Autodesk Inventor part; units mm, degrees
ref_plane "YZ Plane" through (0, 0, 0) normal (1, 0, 0) x (0, 1, 0)
ref_plane "XZ Plane" through (0, 0, 0) normal (0, 1, 0) x (-1, 0, 0)
ref_plane "XY Plane" through (0, 0, 0) normal (0, 0, 1) x (1, 0, 0)
sketch "Skizze1" plane through (0, 0, 0) normal (0, 1, 0) x (-1, 0, 0)
  line L0 (0, 0) -> (0, 79.9753) construction
  line L1 (0, 0) -> (-80.4332, 0) construction
  line L2 (0, 0) -> (80.1339, 0) construction
  line L3 (0, 0) -> (0, -79.3949) construction
  line L4 (0, 1.55) -> (-17, 1.55)
  line L5 (-17, 1.55) -> (-17, 2.95)
  line L6 (-17, 2.95) -> (0, 2.95)
  arc A0 (-1.3565, 0.75) -> (0, 1.55) centre (0, 0) ccw
  arc A1 (-2.8531, 0.75) -> (0, 2.95) centre (0, 0) ccw
  line L7 (-1.3565, 0.75) -> (-2.8531, 0.75)
  circle A2 centre (0, 0) radius 1.5
  dimension "d0" = 1.4
  dimension "d1" = 5.9
  dimension "d2" = 0.8
  dimension "d3" = 19.95
  dimension "d21" = 0.05
  dimension "d28" = 17
extrude "Extrusion1" add sketch "Skizze1" along normal mid plane 60 contours L4 L5 L6 A1 L7 A0
sketch "Skizze3" plane through (0, 0, 0) normal (0, 0, 1) x (1, 0, 0)
  line L0 (7.5, -7.25) -> (-7, -7.25)
  line L1 (-7, -7.25) -> (-7, 7.25)
  line L2 (-7, 7.25) -> (7.5, 7.25)
  line L3 (7.5, 7.25) -> (7.5, -7.25)
  line L4 (17, 30) -> (17, -30) construction
  line L5 (-11.8, 0) -> (21.8, 0) construction
  line L6 (-7, -7.25) -> (5, -7.25)
  line L7 (5, -7.25) -> (5, -21.75)
  line L8 (5, -21.75) -> (-7, -21.75)
  line L9 (-7, -21.75) -> (-7, -7.25)
  line L10 (-7, 7.25) -> (5, 7.25)
  line L11 (5, 7.25) -> (5, 21.75)
  line L12 (5, 21.75) -> (-7, 21.75)
  line L13 (-7, 21.75) -> (-7, 7.25)
  point P0 (0, 0)
  dimension "d6" = 9.5
  dimension "d7" = 14.5
  dimension "d8" = 7.25
  dimension "d9" = 14.5
  dimension "d27" = 12
extrude "Extrusion2" cut sketch "Skizze3" along normal through all both and the other way through all contours L7 L8 L9 L0 | L2 L13 L12 L11
sketch "Skizze4" plane through (17, 30, 1.55) normal (0, 0, -1) x (-1, 0, 0)
  line L0 (17, -72) -> (17, 12)
  line L1 (-3.99, -30) -> (23.94, -30) construction
  line L2 (5, -7.5) -> (5, -52.5) construction
  line L3 (0, 0) -> (0, -60) construction
  point P0 (17, -30)
  point P1 (5, -30)
  dimension "d12" = 45
  dimension "d13" = 5
hole "Bohrung1" at (12, 22.5, 1.55) at (12, -22.5, 1.55) at (12, 0, 1.55) direction (0, 0, 1) diameter 3 end through all countersink diameter 4 countersink angle 90
extrude "Extrusion3" [suppressed]
chamfer "Fase1" [suppressed]
equation "\"d8\" = 0.5 * d7"
equation "\"d9\" = d7"
Geometry check sheet. Reference: the model listing, model coordinates, mm. A direction names the side the tool comes from. Give positions to 0.01 mm unless a question says otherwise; leave off trailing zeros. Loops run counter-clockwise (first coordinate to the right, second up) from the corner with the lowest first, then second, coordinate; pieces in that order, holes last.
(1) Section check A-A on y = 0. Record the cut outline in (x, z).
From the geometry:
outline: (0, 1.55) - (10, 1.55) - (10.5, 2.05) - (10.5, 2.95) - (0, 2.95) arc R2.95 ccw (long way) to (2.85, 0.75) - (1.36, 0.75) arc R1.55 cw (long way) to start; (13.5, 2.05) - (14, 1.55) - (17, 1.55) - (17, 2.95) - (13.5, 2.95) - close
(2) Depth check by flat-ended pin: pin 1 Ø1.1 at (y, z) = (16.5, 2) entering from -X; pin 2 Ø3.5 at (x, y) = (12, -22.5) entering from -Z; pin 3 Ø8.5 at (x, y) = (11.5, -8.5) entering from -Z. Enter the tip coordinate at first touch or a pass-through.
From the geometry:
pin 1: stops at x = 5
pin 2: stops at z = 1.8
pin 3: stops at z = 1.55
(3) Section check C-C on z = -0.3. Record the cut outline in (x, y).
From the geometry:
outline: (-2.93, -30) - (-1.52, -30) - (-1.52, -21.75) - (-2.93, -21.75) - close; (-2.93, -7.25) - (-1.52, -7.25) - (-1.52, 7.25) - (-2.93, 7.25) - close; (-2.93, 21.75) - (-1.52, 21.75) - (-1.52, 30) - (-2.93, 30) - close; (1.52, -30) - (2.93, -30) - (2.93, -21.75) - (1.52, -21.75) - close; (1.52, -7.25) - (2.93, -7.25) - (2.93, 7.25) - (1.52, 7.25) - close; (1.52, 21.75) - (2.93, 21.75) - (2.93, 30) - (1.52, 30) - close
(4) Thickness scan on L1, parallel to Y at x = 12, z = 2.6; L2, parallel to Z at x = 0, y = -26.5; L3, parallel to X at y = 22, z = 0.15. Record the ranges inside material, lowest first.
From the geometry:
L1: y = -30 to -24, -21 to -1.5, 1.5 to 21, 24 to 30
L2: z = -2.95 to -1.55, 1.55 to 2.95
L3: x = -2.95 to -1.54, 1.54 to 2.95
(5) Release check for a two-part mould opening along X. For faces 1 (the cylindrical face through (-1.882, -25.933, -2.272)), 2 (the cylindrical face through (-0.836, -25.933, -1.306)), 3 (the flat face through (2, 26, 0.75)) record: released by +X, released by -X, zero draft, split by the parting line, or undercut.
From the geometry:
face 1: split by the parting line
face 2: undercut
face 3: zero draft
(6) Section check D-D on x = 12. Record the cut outline in (y, z).
From the geometry:
outline: (-30, 1.55) - (-24.5, 1.55) - (-24, 2.05) - (-24, 2.95) - (-30, 2.95) - close; (-21, 2.05) - (-20.5, 1.55) - (-2, 1.55) - (-1.5, 2.05) - (-1.5, 2.95) - (-21, 2.95) - close; (1.5, 2.05) - (2, 1.55) - (20.5, 1.55) - (21, 2.05) - (21, 2.95) - (1.5, 2.95) - close; (24, 2.05) - (24.5, 1.55) - (30, 1.55) - (30, 2.95) - (24, 2.95) - close
(7) Section check B-B on x = 3.5. Record the cut outline in (y, z), then the cut area to 3 significant figures.
From the geometry:
outline: (-30, 1.55) - (-21.75, 1.55) - (-21.75, 2.95) - (-30, 2.95) - close; (-7.25, 1.55) - (7.25, 1.55) - (7.25, 2.95) - (-7.25, 2.95) - close; (21.75, 1.55) - (30, 1.55) - (30, 2.95) - (21.75, 2.95) - close
area: 43.4 mm2
(8) Set-up check for faces 4 (the flat face through (2, -26, 0.75)), 5 (the flat face through (9, 0, 2.95)), 6 (the flat face through (5, -14, 2)): record each of +Z, -Z, +X, -X, +Y, -Y from which the full face is reachable in a straight line by a thin tool's end or side.
From the geometry:
face 4: +X, +Y, -Y
face 5: +Z, +X, -X, +Y, -Y
face 6: +Z, -Z, -X
